from build123d import *

# Parameters (mm, degrees)
SKETCH11_W         = 69.85
SKETCH11_H         = 22.225
SKETCH11_R         = 3.19405
SKETCH11_R_2       = 4.76885
EXTRUDE3_DEPTH     = 7.9375
CUT_EXTRUDE1_DEPTH = 14.3002
FILLET1_R          = 6.35
EXTRUDE4_DEPTH     = 3.9878
SKETCH15_R         = 15.311270849
CUT_EXTRUDE2_DEPTH = 9.001


with BuildPart() as part:
    # Sketch11 → Extrude3 (new body, symmetric)
    with BuildSketch(Plane.XY):
        with Locations((-28.575, 4.7625)):
            Rectangle(SKETCH11_W, SKETCH11_H)
        Circle(SKETCH11_R, mode=Mode.SUBTRACT)
        with Locations((-28.575, 3.175)):
            Circle(SKETCH11_R_2, mode=Mode.SUBTRACT)
    extrude(amount=EXTRUDE3_DEPTH, both=True)

    # Sketch12 → Cut-Extrude1 (cut)
    with BuildSketch(Plane.XZ.offset(6.35)):
        with BuildLine():
            Line((-7.9248, 4.0894), (6.35, 4.0894))
            Line((6.35, 4.0894), (6.35, -4.0894))
            Line((6.35, -4.0894), (-7.9248, -4.0894))
            ThreePointArc((-7.9248, -4.0894), (-12.0142, 0), (-7.9248, 4.0894))
        make_face()
    extrude(amount=-CUT_EXTRUDE1_DEPTH, mode=Mode.SUBTRACT)

    # Fillet1
    fillet1_edges = [part.edges().sort_by_distance(p)[0] for p in [
        (6.35, -6.35, -6.01345),
        (6.35, 15.875, 0),
        (6.35, -6.35, 6.01345),
    ]]
    fillet(fillet1_edges, radius=FILLET1_R)

    # Sketch13 → Extrude4 (add)
    with BuildSketch(Plane(origin=(0, 15.875, 0), x_dir=(1, 0, 0), z_dir=(0, 1, 0))):
        Polygon((-49.641675219, 0), (-53.39583761, 6.5024), (-60.90416239, 6.5024), (-64.658324781, 0), (-60.90416239, -6.5024), (-53.39583761, -6.5024), align=None)
    extrude(amount=EXTRUDE4_DEPTH)

    # Sketch14 → Revolve2 (revolve)
    with BuildSketch(Plane.XY):
        with BuildLine():
            Line((-60.4012, 33.02), (-60.4012, 35.2806))
            Line((-60.4012, 35.2806), (-57.15, 35.2806))
            Line((-57.15, 35.2806), (-57.15, -14.986))
            ThreePointArc((-57.15, -14.986), (-65.618148204, -13.085052733), (-72.461270849, -7.747))
            Line((-72.461270849, -7.747), (-72.461270849, -6.985))
            Line((-72.461270849, -6.985), (-61.1505, -6.985))
            Line((-61.1505, -6.985), (-61.1505, 32.2707))
            Line((-61.1505, 32.2707), (-60.4012, 33.02))
        make_face()
    revolve(axis=Axis((-57.15, 48.481677569, 0), (0, -1, 0)))

    # Sketch15 → Cut-Extrude2 (cut, through all)
    with BuildSketch(Plane(origin=(0, -6.985, 0), x_dir=(1, 0, 0), z_dir=(0, 1, 0))):
        with Locations((-57.15, 0)):
            Circle(SKETCH15_R)
        Polygon((-57.15, 5.657561356), (-62.807561356, 0), (-57.15, -5.657561356), (-51.492438644, 0), align=None, mode=Mode.SUBTRACT)
    extrude(amount=-CUT_EXTRUDE2_DEPTH, mode=Mode.SUBTRACT)


solid = part.part
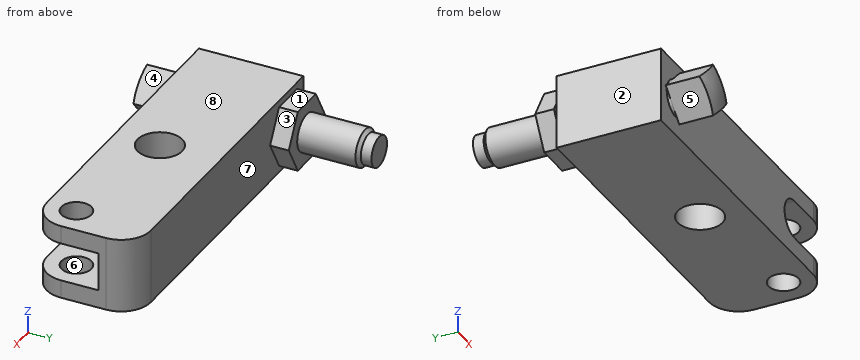
Read the model definition and answer for the solid it produces. Units are mm, in the model's axes. Face numbers are marked on the shaded views. A direction names the side the tool comes from. Give positions to 0.01 mm unless a question says otherwise; leave off trailing zeros. Write each loop counter-clockwise with the first axis right and the second up, starting at its lowest first coordinate (ties: lowest second). Pieces come first, ordered by that corner, then holes. Notation, with made-up numbers: (-32, 77) - (10, 77) arc R29 cw to (10, 102) - close; hole circle Ø8 at (-30.5, 64). An arc over 180 degrees is marked (long way). Use CSV: the item, a comma, the result in double quotes. Start each with the question number.
(1) Find section A-A (y = 18). Give the vertices of the cut face in (x, z).
(2) Find section D-D (y = 11). Give the vertices of the cut face in (x, z), plus the area to 3 significant figures.
(3) Consider line 1 along X through (y, z) = (0, -6.3); line 2 along Y through (x, z) = (0, 6.7) (3 decimals); line 3 along Y through (x, z) = (-46, 1.25) (3 decimals). Determine where each line is inside the solid, lowest interval first.
(4) Determine the mould class of the marked faces 6, 7 and 8 for opening direction Y: +Y half, -Y half, draft (parallel to the pull), parting line (faces both ways), or undercut.
(5) Find section C-C (y = 25.5). Give the vertices of the cut face in (x, z).
(6) For the marked faces 1, 2, 3, 4 and 5, determine the directions among +Z, -Z, +X, -X, +Y, -Y from which every point of the face is accessible in a straight line to the end or side of a thin tool.
(7) Given P1, Ø1, axis at x = -50.5, z = 3, coming from the -Y side; P2, Ø3, axis at x = -6.5, z = 0, coming from the -Y side; P3, Ø1.4, axis at x = -56.5, z = 4, coming from the +Y side, each flat-ended and moving along its own axis, determine where each tip first touches the part or whether it passes through.
Findings below:
1,outline,"(-64.66, 0) - (-60.9, -6.5) - (-53.4, -6.5) - (-49.64, 0) - (-53.4, 6.5) - (-60.9, 6.5) - close"
2,outline,"(-63.5, -7.94) - (6.18, -7.94) - (6.18, 7.94) - (-63.5, 7.94) - close"
2,area,"1,110 mm2"
3,line 1,"-63.5 to -32.13, -25.02 to -3.19, 3.19 to 6.35"
3,line 2,"-6.35 to -3.194, 3.194 to 15.875"
3,line 3,"-6.35 to 15.875"
4,face 6,"undercut"
4,face 7,"+Y half"
4,face 8,"draft"
5,outline,"circle Ø8 at (-57.15, 0)"
6,face 1,"+Z, +X, -X, +Y"
6,face 2,"+Z, -Z, -X, -Y"
6,face 3,"+Z, +X, +Y"
6,face 4,"+Z, +X, -Y"
6,face 5,"-Z, -X, -Y"
7,P1,"y = -6.35"
7,P2,"y = 7.95"
7,P3,"y = 32.92"
